Verification items for the finished model (mm, model axes). Face numbers are marked on the shaded views. A direction names the side the tool comes from. Round coordinates to 2 decimals unless told otherwise and drop trailing zeros. Order: outer loops, then holes, each group sorted by start corner. A loop starts at its lowest first (then second) coordinate and runs counter-clockwise, first axis right, second up. Notation, with made-up numbers: (47.25, 10) -> (87.25, 10) arc R32 cw to (87.25, 48) -> close; hole circle Ø7 at (-22, 13). An arc over 180 degrees is marked (long way). Return JSON: item names as keys, results as strings. Group by question number.
Item 1: Scan lines: probe 1 along Z at (x, y) = (8, 16.5); probe 2 along X at (y, z) = (3.5, 16.5); probe 3 along X at (y, z) = (21, 56). Record each from-to range of solid material in increasing order. Write a range as from..to.
Item 2: Depth check by flat-ended pin: pin 1 Ø3 at (x, z) = (13.5, 12) entering from +Y; pin 2 Ø16.5 at (y, z) = (11.5, 35.5) entering from +X; pin 3 Ø9 at (x, z) = (-42.5, 56) entering from +Y; pin 4 Ø12 at (y, z) = (64.5, 8) entering from -X. Enter the tip coordinate at first touch or a pass-through.
Item 3: Draft check along Z on the marked faces 1, 2 and 3. Enter one of: pulls with the +Z half, pulls with the -Z half, needs draft (parallel to the pull), parting line crosses it, or undercut.
Item 4: Sectioned sample at B-B on z = 17.5. Record the cut outline in (x, y).
Item 5: Sectioned sample at C-C on x = 0. Record the cut outline in (y, z), plus the area to 3 significant figures.
Item 6: Access from +Z, -Z, +X, -X, +Y, -Y to the whole of each face (thin tool, end or side, straight path). Record for the marked faces 4, 5, 6 and 7.
Item 7: Sectioned sample at D-D on z = 57. Record the cut outline in (x, y), plus the area to 3 significant figures.
Item 8: Sectioned sample at A-A on y = 10.5. Record the cut outline in (x, z), plus the area to 3 significant figures.
```python
from build123d import *

# Parameters (mm, degrees)
SKETCH1_W           = 80
SKETCH1_H           = 70
BOSS_EXTRUDE1_DEPTH = 15
BOSS_EXTRUDE2_DEPTH = 70
BOSS_EXTRUDE3_DEPTH = 15
BOSS_EXTRUDE4_DEPTH = 20
CUT_EXTRUDE1_DEPTH  = 116.758369028
SKETCH6_W           = 40
SKETCH6_H           = 40
CUT_EXTRUDE2_DEPTH  = 116.758369028


with BuildPart() as part:
    # Sketch1 → Boss-Extrude1 (new body)
    with BuildSketch(Plane(origin=(0, 0, 0), x_dir=(1, 0, 0), z_dir=(0, 1, 0))):
        with Locations((0, -35)):
            Rectangle(SKETCH1_W, SKETCH1_H)
    extrude(amount=BOSS_EXTRUDE1_DEPTH)

    # Sketch2 → Boss-Extrude2 (add)
    with BuildSketch(Plane.XY):
        with BuildLine():
            Line((-30, 10), (30, 10))
            Line((30, 10), (30, 28.542486889))
            ThreePointArc((30, 28.542486889), (37.416573868, 40.857864376), (40, 55))
            Line((40, 55), (-40, 55))
            ThreePointArc((-40, 55), (-37.416573868, 40.857864376), (-30, 28.542486889))
            Line((-30, 28.542486889), (-30, 10))
        make_face()
    extrude(amount=BOSS_EXTRUDE2_DEPTH)

    # Sketch3 → Boss-Extrude3 (add)
    with BuildSketch(Plane(origin=(0, 0, 0), x_dir=(1, 0, 0), z_dir=(0, 1, 0))):
        Polygon((-60, 0), (-38, 0), (-38, -70), (-40, -70), (-60, -20), align=None)
    boss_extrude3 = extrude(amount=BOSS_EXTRUDE3_DEPTH)

    # Sketch4 → Boss-Extrude4 (add)
    with BuildSketch(Plane.XY):
        Polygon((-60, 15), (-30, 15), (-30, 70), (-40, 70), align=None)
    boss_extrude4 = extrude(amount=BOSS_EXTRUDE4_DEPTH)

    # Mirror1: Boss-Extrude3, Boss-Extrude4 across plane
    add(boss_extrude3.mirror(Plane(origin=(0, 0, 0), x_dir=(0, 0, 1), z_dir=(1, 0, 0))))
    add(boss_extrude4.mirror(Plane(origin=(0, 0, 0), x_dir=(0, 0, 1), z_dir=(1, 0, 0))))

    # Sketch5 → Cut-Extrude1 (cut, through all)
    with BuildSketch(Plane.XY):
        with BuildLine():
            Line((-30, 55), (30, 55))
            ThreePointArc((30, 55), (0, 25), (-30, 55))
        make_face()
    extrude(amount=CUT_EXTRUDE1_DEPTH, mode=Mode.SUBTRACT)

    # Sketch6 → Cut-Extrude2 (cut, through all)
    with BuildSketch(Plane(origin=(0, 0, 0), x_dir=(1, 0, 0), z_dir=(0, 1, 0))):
        with Locations((0, -30)):
            Rectangle(SKETCH6_W, SKETCH6_H)
    extrude(amount=CUT_EXTRUDE2_DEPTH, mode=Mode.SUBTRACT)


solid = part.part
```
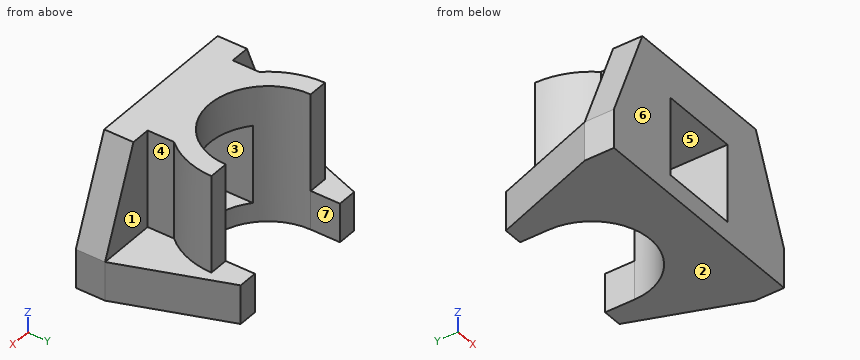
Recorded:
{
 "1": {"probe 1": "0..10, 50..70", "probe 2": "-60..-20, 20..60", "probe 3": "-30..30"},
 "2": {"pin 1": "through", "pin 2": "x = 57.1", "pin 3": "y = 55", "pin 4": "x = -44.18"},
 "3": {"face 1": "needs draft", "face 2": "pulls with the -Z half", "face 3": "undercut"},
 "4": {"outline": "(-60, 0) -> (-20, 0) -> (-20, 32.64) arc R30 cw to (-30, 55) -> (-30, 70) -> (-40, 70) -> (-60, 15) -> close; (20, 0) -> (60, 0) -> (60, 15) -> (40, 70) -> (30, 70) -> (30, 55) arc R30 cw to (20, 32.64) -> close"},
 "5": {"outline": "(0, 0) -> (25, 0) -> (25, 10) -> (0, 10) -> close; (0, 50) -> (25, 50) -> (25, 70) -> (0, 70) -> close", "area": "750 mm²"},
 "6": {"face 4": "+Z, +X", "face 5": "+Y, -Y", "face 6": "+Z, -Z, +X, -X, -Y", "face 7": "+Z, -Z, +Y"},
 "7": {"outline": "(-45.2, 0) -> (45.2, 0) -> (45.2, 15) -> (30, 15) -> (30, 28.54) arc R40 ccw to (40, 55) -> (30, 55) arc R30 cw to (-30, 55) -> (-40, 55) arc R40 ccw to (-30, 28.54) -> (-30, 15) -> (-45.2, 15) -> close", "area": "2,700 mm²"},
 "8": {"outline": "(-60, 0) -> (60, 0) -> (60, 20) -> (40, 70) -> (-40, 70) -> (-60, 20) -> close; hole (-20, 10) -> (20, 10) -> (20, 50) -> (-20, 50) -> close", "area": "5,800 mm²"}
}
